Geometry check sheet. Reference: the model listing, model coordinates, mm. Round coordinates to 2 decimals unless told otherwise and drop trailing zeros. Write each loop counter-clockwise with the first axis right and the second up, starting at its lowest first coordinate (ties: lowest second). Pieces come first, ordered by that corner, then holes. Notation, with made-up numbers: M 82.5,1 L 113.5,1 A23 ccw 113.5,28 Z; hole C 23.25,-23 d8. An arc over 180 degrees is marked long. Use a Markdown table: item, result.
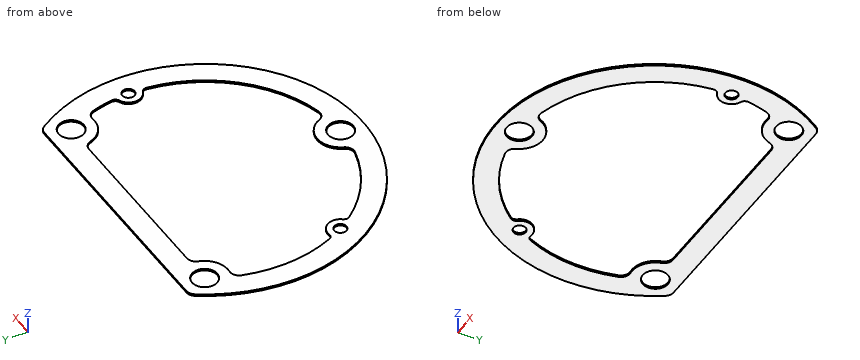
```python
from build123d import *

# Parameters (mm, degrees)
SKETCH_1_R      = 7
EXTRUDE_1_DEPTH = 1
SKETCH_2_R      = 3.75
SKETCH_3_R      = 3
SKETCH_2_4_R    = 3.75
SKETCH_3_4_R    = 3


with BuildPart() as part:
    # Эскиз1 → Бобышка-Вытянуть1 (new body)
    with BuildSketch(Plane.XY):
        with BuildLine():
            Line((-69.14658343, 50), (69.14658343, 50))
            ThreePointArc((69.14658343, 50), (71.530239903, 49.395245365), (73.337285456, 47.727272727))
            ThreePointArc((73.337285456, 47.727272727), (0, -87.5), (-73.337285456, 47.727272727))
            ThreePointArc((-73.337285456, 47.727272727), (-71.530239903, 49.395245365), (-69.14658343, 50))
        make_face()
        with Locations((-64.95, 37.503299855)):
            Circle(SKETCH_1_R, mode=Mode.SUBTRACT)
        with Locations((64.95, 37.503299855)):
            Circle(SKETCH_1_R, mode=Mode.SUBTRACT)
        with Locations((0, -75)):
            Circle(SKETCH_1_R, mode=Mode.SUBTRACT)
        with BuildLine():
            Line((-47.658383534, 37.503299855), (47.658383534, 37.503299855))
            ThreePointArc((47.658383534, 37.503299855), (50.663009597, 36.499826124), (52.46161033, 33.892188744))
            ThreePointArc((52.46161033, 33.892188744), (57.800209242, 26.646021554), (66.56595151, 24.604125435))
            ThreePointArc((66.56595151, 24.604125435), (69.931223097, 23.822835867), (71.986576416, 21.045969112))
            ThreePointArc((71.986576416, 21.045969112), (73.39628095, 15.426793015), (74.368055556, 9.715570641))
            ThreePointArc((74.368055556, 9.715570641), (73.972679073, 7.794963627), (72.475333333, 6.528863471))
            ThreePointArc((72.475333333, 6.528863471), (68, 0), (72.475333333, -6.528863471))
            ThreePointArc((72.475333333, -6.528863471), (73.972679073, -7.794963627), (74.368055556, -9.715570641))
            ThreePointArc((74.368055556, -9.715570641), (55.850918931, -50.056716378), (17.770646228, -72.864285714))
            ThreePointArc((17.770646228, -72.864285714), (14.338112526, -72.472905294), (11.978731902, -69.949259259))
            ThreePointArc((11.978731902, -69.949259259), (0, -62), (-11.978731902, -69.949259259))
            ThreePointArc((-11.978731902, -69.949259259), (-14.338112526, -72.472905294), (-17.770646228, -72.864285714))
            ThreePointArc((-17.770646228, -72.864285714), (-40.749625279, -62.964021787), (-59.19327098, -46.056016661))
            ThreePointArc((-59.19327098, -46.056016661), (-59.825507849, -44.199856536), (-59.176073891, -42.349643196))
            ThreePointArc((-59.176073891, -42.349643196), (-58.625658395, -34.453333333), (-65.791988875, -31.092027915))
            ThreePointArc((-65.791988875, -31.092027915), (-67.724404324, -30.759124925), (-69.038382563, -29.303612969))
            ThreePointArc((-69.038382563, -29.303612969), (-74.871756142, -4.384077128), (-71.986576416, 21.045969112))
            ThreePointArc((-71.986576416, 21.045969112), (-69.931223097, 23.822835867), (-66.56595151, 24.604125435))
            ThreePointArc((-66.56595151, 24.604125435), (-57.800209242, 26.646021554), (-52.46161033, 33.892188744))
            ThreePointArc((-52.46161033, 33.892188744), (-50.663009597, 36.499826124), (-47.658383534, 37.503299855))
        make_face(mode=Mode.SUBTRACT)
    extrude(amount=EXTRUDE_1_DEPTH)

    # Эскиз2 → Вырез-По сечениям1 section 0
    with BuildSketch(Plane(origin=(0, 0, -18), x_dir=(-1, 0, 0), z_dir=(0, 0, -1))):
        with Locations((64.660652641, -38)):
            Circle(SKETCH_2_R)
    # Эскиз3 → Вырез-По сечениям1 section 1
    with BuildSketch(Plane.XY.offset(25)):
        with Locations((-64.660652641, -38)):
            Circle(SKETCH_3_R)
    loft(mode=Mode.SUBTRACT)

    # Эскиз2<4> → Вырез-По сечениям2 section 0
    with BuildSketch(Plane(origin=(0, 0, -18), x_dir=(-1, 0, 0), z_dir=(0, 0, -1))):
        with Locations((-75, 0)):
            Circle(SKETCH_2_4_R)
    # Эскиз3<4> → Вырез-По сечениям2 section 1
    with BuildSketch(Plane.XY.offset(25)):
        with Locations((75, 0)):
            Circle(SKETCH_3_4_R)
    loft(mode=Mode.SUBTRACT)


solid = part.part
```
Item 1: Go/stop test with a flat-tipped pin: pin 1 (11 mm diameter, centred on x = 64.95, y = 37.5, fed in from +Z). Record where the tip stops, or that it passes through.
Outcome:
| item | result |
|---|---|
| pin 1 | passes through |
Item 2: Material ranges on line 1 along Y through (x, z) = (0, 0.85); line 2 along Y through (x, z) = (-64.95, 0.55); line 3 along Y through (x, z) = (-22, 0.4), recorded low to high. Write a range as from..to.
Outcome:
| item | result |
|---|---|
| line 1 | y = -87.5..-82, -68..-62, 37.5..50 |
| line 2 | y = -58.63..-41.41, -34.59..-31.01, 24.5..30.5, 44.5..50 |
| line 3 | y = -84.69..-71.7, 37.5..50 |
Item 3: Cross-section at C-C, the plane z = 0.5. Count the separate pieces of the cut face and the enclosed holes in it, and give its area (3 significant figures).
Outcome:
| item | result |
|---|---|
| separate pieces | 1 |
| enclosed holes | 6 |
| area | 6,300 mm2 |
Item 4: Cross-section at A-A, the plane x = 49.5. Record the cut outline in (y, z).
Outcome:
| item | result |
|---|---|
| outline | M -72.15,0 L -56.34,0 L -56.34,1 L -72.15,1 Z; M 37.15,0 L 50,0 L 50,1 L 37.15,1 Z |
Item 5: Cross-section at B-B, the plane y = -60. Record the cut outline in (x, z).
Outcome:
| item | result |
|---|---|
| outline | M -63.69,0 L -45,0 L -45,1 L -63.69,1 Z; M 45,0 L 63.69,0 L 63.69,1 L 45,1 Z |
